Design review of the part built by this model. Coordinates are the model's own, in mm. Face numbers are marked on the shaded views. A direction names the side the tool comes from. Coordinates: 2 decimals unless noted, no trailing zeros. Loops run counter-clockwise (first coordinate to the right, second up) from the corner with the lowest first, then second, coordinate; pieces in that order, holes last. Notation, with made-up numbers: (31.25, -18) - (78.25, -18) arc R18 ccw to (78.25, 15) - close; hole circle Ø9 at (83, 56). An arc over 180 degrees is marked (long way). Return JSON: item names as keys, results as strings. Group by question number.
from build123d import *

# Parameters (mm, degrees)
F0_W     = 20
F0_H     = 28.9
F1_DEPTH = 8
F2_W     = 9
F2_H     = 4.5
F3_DEPTH = 28.901
F5_D     = 3.2
F5_DEPTH = 4
F5_TIP   = 0.9613769904


with BuildPart() as f1:
    # F0 (on Top) → F1 (new body)
    with BuildSketch(Plane.XY):
        with Locations((10, 14.45)):
            Rectangle(F0_W, F0_H)
    extrude(amount=F1_DEPTH)

    # F2 (on face) → F3 (cut, through all)
    with BuildSketch(Plane.XZ):
        with Locations((10, 2.25)):
            Rectangle(F2_W, F2_H)
    extrude(amount=-F3_DEPTH, mode=Mode.SUBTRACT)

    # F5
    with Locations(Plane.XY.offset(8)):
        with Locations((2.5, 9.45), (2.5, 19.45), (17.5, 19.45), (17.5, 9.45)):
            Hole(F5_D / 2, depth=F5_DEPTH)
            with Locations((0, 0, -(F5_DEPTH + F5_TIP / 2))):  # 118° drill point
                Cone(0, F5_D / 2, F5_TIP, mode=Mode.SUBTRACT)


solid = f1.part
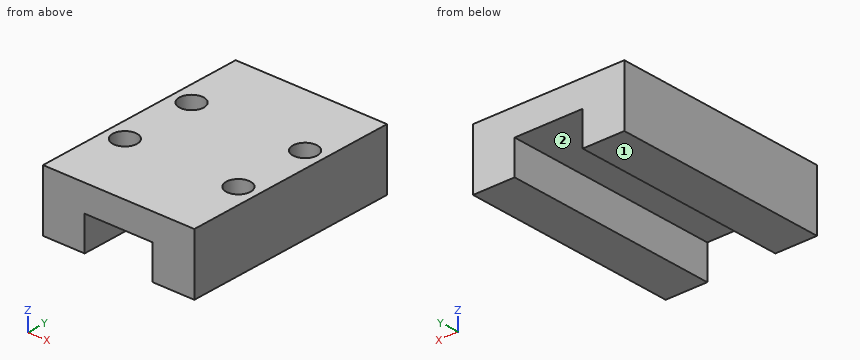
Item 1: Add section B-B (z = 5). State the section outline as (x, y) points, then the cut area to 3 significant figures.
Item 2: To check wall thickness, follow line 1 (Y direction, x = 2.5, z = 4.95); line 2 (X direction, y = 9.45, z = 5.05); line 3 (X direction, y = 16.5, z = 1.25). State the ranges of each line that lie inside material, in increasing order. Write a range as from..to.
Item 3: For P1, Ø2.5, axis at x = 17.5, y = 19.45, coming from the +Z side; P2, Ø3, axis at x = 12.5, z = 1.5, coming from the +Y side, all flat-tipped, find the tip position at first contact; note any pin that passes through.
Item 4: Add section C-C (y = 7.5). State the section outline as (x, z) points.
Item 5: Add section A-A (z = 2.25). State the section outline as (x, y) points.
Item 6: For the marked faces 1 and 2, list the 3-axis set-ups (+Z, -Z, +X, -X, +Y, -Y) from which the entire face can be reached by the end or side of a thin tool; tool diameter is ignored.
Answers below:
{
 "1": {"outline": "(0, 0) - (20, 0) - (20, 28.9) - (0, 28.9) - close; hole circle Ø3.2 at (2.5, 9.45); hole circle Ø3.2 at (2.5, 19.45); hole circle Ø3.2 at (17.5, 9.45); hole circle Ø3.2 at (17.5, 19.45)", "area": "546 mm^2"},
 "2": {"line 1": "y = 0..7.85, 11.05..17.85, 21.05..28.9", "line 2": "x = 0..0.9, 4.1..15.9, 19.1..20", "line 3": "x = 0..5.5, 14.5..20"},
 "3": {"P1": "stops at z = 3.79", "P2": "passes through"},
 "4": {"outline": "(0, 0) - (5.5, 0) - (5.5, 4.5) - (14.5, 4.5) - (14.5, 0) - (20, 0) - (20, 8) - (0, 8) - close"},
 "5": {"outline": "(0, 0) - (5.5, 0) - (5.5, 28.9) - (0, 28.9) - close; (14.5, 0) - (20, 0) - (20, 28.9) - (14.5, 28.9) - close"},
 "6": {"face 1": "-Z, +X, -X, +Y, -Y", "face 2": "-Z, +Y, -Y"}
}
